from build123d import *

# Parameters (mm, degrees)
F0_W     = 100
F0_H     = 40
F1_DEPTH = 50
F2_R     = 15
F3_DEPTH = 10
F4_W     = 90
F4_H     = 30
F5_DEPTH = 40


with BuildPart() as f1:
    # F0 (on Top) → F1 (new body)
    with BuildSketch(Plane.XY):
        Rectangle(F0_W, F0_H)
    extrude(amount=F1_DEPTH)

    # F2 (on face) → F3 (join)
    with BuildSketch(Plane.XY.offset(50)):
        with Locations((30, 0)):
            Circle(F2_R)
        with Locations((-30, 0)):
            Circle(F2_R)
    extrude(amount=F3_DEPTH)

    # F4 (on face) → F5 (cut)
    with BuildSketch(Plane(origin=(0, 0, 0), x_dir=(1, 0, 0), z_dir=(0, 0, -1))):
        Rectangle(F4_W, F4_H)
    extrude(amount=-F5_DEPTH, mode=Mode.SUBTRACT)


solid = f1.part
CAD build for the part. Positions are in the model's coordinates, mm. A direction names the side the tool comes from. Round coordinates to 2 decimals unless told otherwise and drop trailing zeros. Write each loop counter-clockwise with the first axis right and the second up, starting at its lowest first coordinate (ties: lowest second). Pieces come first, ordered by that corner, then holes. Notation, with made-up numbers: M -4.75,-29.75 L 34.25,-29.75 A14 cw 34.25,-20.75 Z; hole C 73.5,45.5 d7. An arc over 180 degrees is marked long. Use a Markdown table: item, result. Add a question column.
1. Slice it at A-A on z = 23. Give the cut face in (x, y).
2. 3-axis set-ups, long thin cutter, end or side, ignore diameter. For faces 4 (the face through (30, 0, 60)), 5 (the face through (-1, -15, 20)), 6 (the face through (15.015, 0.66, 54.93)): which of +Z, -Z, +X, -X, +Y, -Y reach the whole face in a straight line?
3. Pull direction X, two halves, no side cores. Call faces 1 (the face through (50, 0, 25)), 2 (the face through (-1, 15, 20)), 3 (the face through (-30, 0, 60)): released by +X, released by -X, zero draft, split by the parting line, or undercut.
4. Slice it at D-D on x = 30.5. Give the cut face in (y, z).
5. Slice it at B-B on y = 0. Give the cut face in (x, z).
6. Flat gauge pins, fed straight in: P1, Ø10, axis at y = -0.5, z = 53.5, coming from the +X side; P2, Ø2, axis at x = -8, y = -3.5, coming from the -Z side. Where does each tip first touch, or does it go through?
7. Slice it at C-C on x = -12. Give the cut face in (y, z), then the cut area to 3 significant figures.
8. Drill centre lines: probe 1 along X at (y, z) = (14.5, 18.5); probe 2 along Y at (x, z) = (7.5, 18); probe 3 along Z at (x, y) = (11.5, 14). Where is each one in solid material? Low to high.
Reply:
| question | item | result |
|---|---|---|
| 1 | outline | M -50,-20 L 50,-20 L 50,20 L -50,20 Z; hole M -45,-15 L 45,-15 L 45,15 L -45,15 Z |
| 2 | face 4 | +Z, +X, -X, +Y, -Y |
| 2 | face 5 | -Z |
| 2 | face 6 | +Z |
| 3 | face 1 | released by +X |
| 3 | face 2 | undercut |
| 3 | face 3 | zero draft |
| 4 | outline | M -20,0 L -15,0 L -15,40 L 15,40 L 15,0 L 20,0 L 20,50 L 14.99,50 L 14.99,60 L -14.99,60 L -14.99,50 L -20,50 Z |
| 5 | outline | M -50,0 L -45,0 L -45,40 L 45,40 L 45,0 L 50,0 L 50,50 L 45,50 L 45,60 L 15,60 L 15,50 L -15,50 L -15,60 L -45,60 L -45,50 L -50,50 Z |
| 6 | P1 | stops at x = 50 |
| 6 | P2 | stops at z = 40 |
| 7 | outline | M -20,0 L -15,0 L -15,40 L 15,40 L 15,0 L 20,0 L 20,50 L -20,50 Z |
| 7 | area | 800 mm^2 |
| 8 | probe 1 | x = -50 to -45, 45 to 50 |
| 8 | probe 2 | y = -20 to -15, 15 to 20 |
| 8 | probe 3 | z = 40 to 50 |
